Source: CAD feature listing. Evaluate the final solid. Frame: model axes, mm. Face numbers are marked on the shaded views. A direction names the side the tool comes from. Coordinates: 2 decimals unless noted, no trailing zeros. Loops run counter-clockwise (first coordinate to the right, second up) from the corner with the lowest first, then second, coordinate; pieces in that order, holes last. Notation, with made-up numbers: (87, -15.75) - (112, -15.75) arc R31 ccw to (112, 14.25) - close; hole circle Ø1 at (-25, 81). An arc over 180 degrees is marked (long way). Use CSV: the item, a comma, the result in double quotes. Start each with the question number.
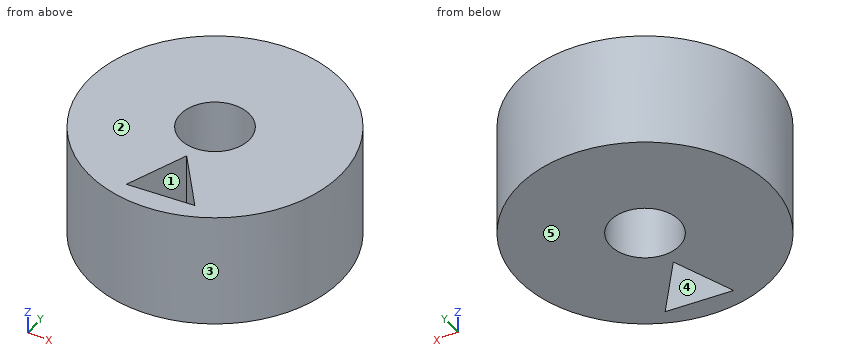
```python
from build123d import *

# Parameters (mm, degrees)
F0_R     = 5.5
F0_R_2   = 1.5
F1_DEPTH = 5
F3_DEPTH = 5


with BuildPart() as f1:
    # F0 (on Top) → F1 (new body)
    with BuildSketch(Plane.XY):
        Circle(F0_R)
        Circle(F0_R_2, mode=Mode.SUBTRACT)
    extrude(amount=F1_DEPTH)

    # F2 (on face) → F3 (cut)
    with BuildSketch(Plane.XY.offset(5)):
        Polygon((1.809749, -4.461624), (0, -2.042668), (-1.033585, -4.673813), align=None)
    extrude(amount=-F3_DEPTH, mode=Mode.SUBTRACT)


solid = f1.part
```
(1) Reachability of the marked faces 1 and 2 from +Z, -Z, +X, -X, +Y, -Y: full face, straight path, thin tool, end or side. Return the list, or none.
(2) Draft query along Y for the marked faces 3, 4 and 5. Return one class per face: released by +Y, released by -Y, zero draft, split by the parting line, or undercut.
(3) Section C-C on x = 2.5. Output: boundary loops of the cut face in (y, z).
(4) Section D-D on y = 2.75. Output: boundary loops of the cut face in (x, z).
(5) Section B-B on z = 1.1. Output: boundary loops of the cut face in (x, y), plus the area to 3 significant figures.
(6) Ray query, line 1 (Y direction, x = 1.25, z = 1.95); line 2 (Y direction, x = 1, z = 2.5); line 3 (X direction, y = -2.25, z = 1.1). Return the intervals inside material, ascending. Write a range as [from, to].
(7) Pin query (flat end, axial travel): pin 1 Ø1.5 at (x, z) = (3, 3.5) entering from +Y; pin 2 Ø3 at (x, z) = (-4.5, 3) entering from -Y. Return the tip coordinate at first contact, or that it passes through.
(8) Section A-A on y = 0. Output: boundary loops of the cut face in (x, z), plus the area to 3 significant figures.
Solution:
1,face 1,"+Z, -Z"
1,face 2,"+Z, +X, -X, +Y, -Y"
2,face 3,"split by the parting line"
2,face 4,"undercut"
2,face 5,"zero draft"
3,outline,"(-4.9, 0) - (4.9, 0) - (4.9, 5) - (-4.9, 5) - close"
4,outline,"(-4.76, 0) - (4.76, 0) - (4.76, 5) - (-4.76, 5) - close"
5,outline,"circle Ø11 at (0, 0); hole circle Ø3 at (0, 0); hole (-1.03, -4.67) - (1.81, -4.46) - (0, -2.04) - close"
5,area,"84.3 mm²"
6,line 1,"y = [-5.36, -4.5], [-3.71, -0.83], [0.83, 5.36]"
6,line 2,"y = [-5.41, -4.52], [-3.38, -1.12], [1.12, 5.41]"
6,line 3,"x = [-5.02, -0.08], [0.16, 5.02]"
7,pin 1,"stops at y = 5.02"
7,pin 2,"stops at y = -4.61"
8,outline,"(-5.5, 0) - (-1.5, 0) - (-1.5, 5) - (-5.5, 5) - close; (1.5, 0) - (5.5, 0) - (5.5, 5) - (1.5, 5) - close"
8,area,"40.0 mm²"
